Build history of the part. All positions in model axes, mm. A direction names the side the tool comes from. Round coordinates to 2 decimals unless told otherwise and drop trailing zeros. Order: outer loops, then holes, each group sorted by start corner. A loop starts at its lowest first (then second) coordinate and runs counter-clockwise, first axis right, second up. Notation, with made-up numbers: M 58.25,40 L 68.25,40 A24 ccw 68.25,62 Z; hole C 7,34.5 d9. An arc over 180 degrees is marked long. One line per item, written item: value. Start each with the question number.
Item 1: Band-saw the part on B-B, the plane y = -156. Write the cut outline in (x, z), then the cut area to 3 significant figures.
Item 2: Band-saw the part on C-C, the plane z = 42. Write the cut outline in (x, y).
Item 3: Tool access for faces 5 (the flat face through (-3, 248, 1)), 6 (the flat face through (-200, -230, 2)), 7 (the flat face through (-3, 45.447, -62)), 8 (the flat face through (200, 245, 2)): list every direction of +Z, -Z, +X, -X, +Y, -Y with a clear straight run to the whole face (end or side of a thin tool).
Item 4: Band-saw the part on D-D, the plane y = 134. Write the cut outline in (x, z), then the cut area to 3 significant figures.
Item 5: Band-saw the part on A-A, the plane x = 23. Write the cut outline in (y, z), then the cut area to 3 significant figures.
Item 6: Two-plate mould, pull along X, no slides. Class faces 1 (the flat face through (-250, -7, 2)), 2 (the flat face through (-2, -224, -1)), 3 (the flat face through (-3, 45.447, 64)), 4 (the flat face through (-3, 7, 125)): +X half, -X half, draft (parallel to the pull), parting line (faces both ways), or undercut.
Item 7: Pin check, flat tips, straight feed: pin 1 (1.5 mm diameter, centred on x = 99.5, y = 99.5, fed in from -Z); pin 2 (1 mm diameter, centred on x = -129.5, y = 195, fed in from +Z). Stop position of each tip, or through.
Item 8: Probe L1, parallel to Y at x = -21.5, z = 27.5; L2, parallel to X at y = -235, z = -104; L3, parallel to Z at x = -53.5, y = -312.5. List the from-to ranges inside material, lowest first.
```python
from build123d import *

# Parameters (mm, degrees)
F0_W     = 500
F0_H     = 1000
F0_W_2   = 400
F0_H_2   = 445.4466052353
F0_H_3   = 404.5533947647
F1_DEPTH = 125
F2_W     = 401.6181921197
F2_H     = 400
F2_W_2   = 400
F2_H_2   = 450
F3_DEPTH = 1


with BuildPart() as f1:
    # F0 (on Top) → F1 (new body, symmetric)
    with BuildSketch(Plane.XY):
        Rectangle(F0_W, F0_H)
        with Locations((0, -227.2766973823)):
            Rectangle(F0_W_2, F0_H_2, mode=Mode.SUBTRACT)
        with Locations((0, 247.7233026177)):
            Rectangle(F0_W_2, F0_H_3, mode=Mode.SUBTRACT)
    extrude(amount=F1_DEPTH, both=True)

    # F2 (on Top) → F3 (join, symmetric)
    with BuildSketch(Plane.XY):
        with Locations((0.8090960599, 245.0032802157)):
            Rectangle(F2_W, F2_H)
        with Locations((1.6181921197, -225)):
            Rectangle(F2_W_2, F2_H_2)
    extrude(amount=F3_DEPTH, both=True)


solid = f1.part
```
Output:
1. outline: M -250,-125 L -200,-125 L -200,125 L -250,125 Z; M -198.38,-1 L 200,-1 L 200,-125 L 250,-125 L 250,125 L 200,125 L 200,1 L -198.38,1 Z
1. area: 25,800 mm²
2. outline: M -250,-500 L 250,-500 L 250,500 L -250,500 Z; hole M -200,-450 L 200,-450 L 200,-4.55 L -200,-4.55 Z; hole M -200,45.45 L 200,45.45 L 200,450 L -200,450 Z
3. face 5: +Z
3. face 6: +Z, -Z
3. face 7: -Z
3. face 8: none
4. outline: M -250,-125 L -200,-125 L -200,-1 L 200,-1 L 200,-125 L 250,-125 L 250,125 L 200,125 L 200,1 L -200,1 L -200,125 L -250,125 Z
4. area: 25,800 mm²
5. outline: M -500,-125 L -450,-125 L -450,-1 L -4.55,-1 L -4.55,-125 L 45.45,-125 L 45.45,-1 L 445,-1 L 445,1 L 45.45,1 L 45.45,125 L -4.55,125 L -4.55,1 L -450,1 L -450,125 L -500,125 Z; M 450,-125 L 500,-125 L 500,125 L 450,125 Z
5. area: 39,200 mm²
6. face 1: -X half
6. face 2: undercut
6. face 3: undercut
6. face 4: draft
7. pin 1: stops at z = -1
7. pin 2: stops at z = 1
8. L1: y = -500 to -450, -4.55 to 45.45, 450 to 500
8. L2: x = -250 to -200, 200 to 250
8. L3: z = -1 to 1
